Here's the drawing with two shaded views (mm, measured from the low corner). I have some questions. Coordinates: 2 decimals unless noted, no trailing zeros. Order: outer loops, then holes, each group sorted by start corner. A loop starts at its lowest first (then second) coordinate and runs counter-clockwise, first axis right, second up. Notation, with made-up numbers: (-37.75, -8) -> (-31.75, -8) arc R23 ccw to (-31.75, 8) -> close; hole circle Ø3 at (24, 89.5). An arc over 180 degrees is marked (long way). Return JSON: item names as keys, results as strings. Group by question number.
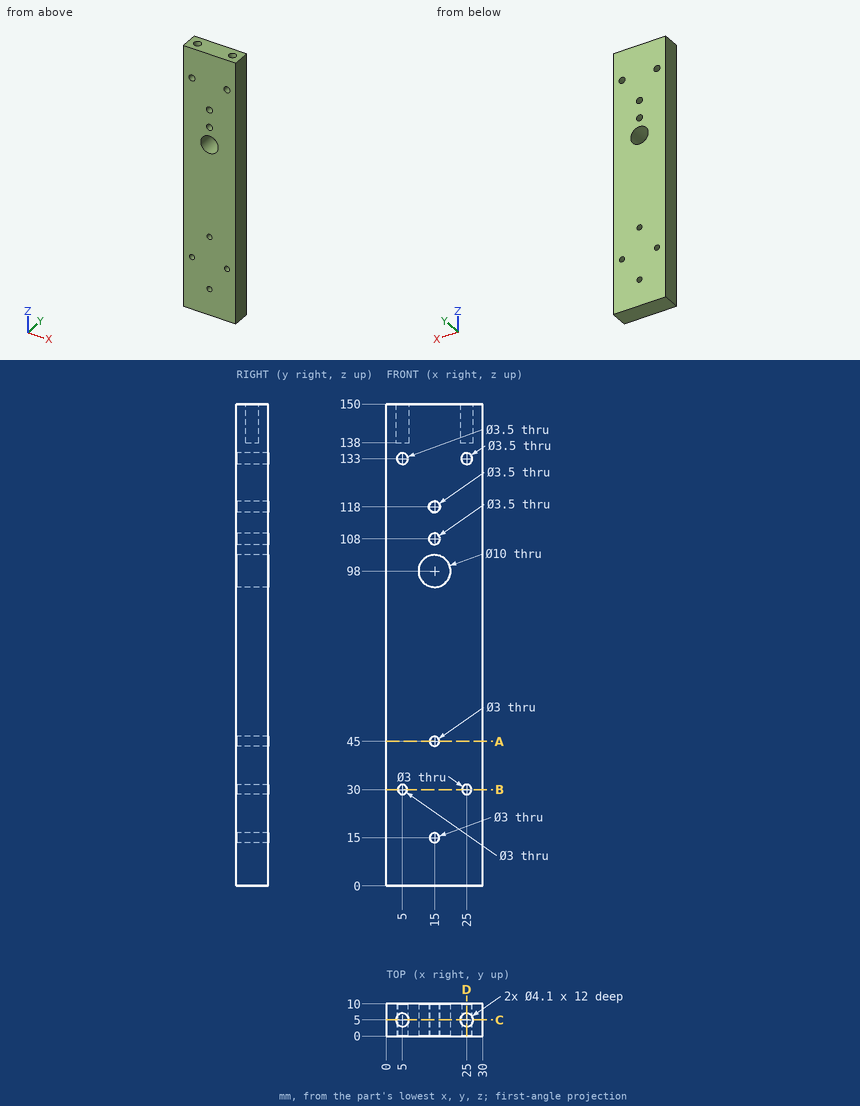
Q1. I'm going to push a flat-ended pin straight in: pin 1 Ø2 at (x, z) = (15, 118) entering from -Y. Where does the tip first touch, or does it pass through?
Q2. I need wall thicknesses on line 1 along Z through (x, y) = (15, 7.75); line 2 along X through (y, z) = (5.5, 133); line 3 along Z through (x, y) = (5, 8). Which ranges of each line are inside material? Lowest first, please. Write a range as from..to.
Q3. I want a section at A-A on z = 45. Please give me the cut outline in (x, y).
Q4. I want a section at C-C on y = 5. State how many separate pieces and enclosed holes the cut face has, and give its area (3 significant figures).
Q5. I want a section at B-B on z = 30. Please give me the cut outline in (x, y), and give its area (3 significant figures).
Q6. I want a section at D-D on x = 25. Please give me the cut outline in (y, z), and give its area (3 significant figures).
Response values:
{
 "1": {"pin 1": "passes through"},
 "2": {"line 1": "z = 0..13.5, 16.5..43.5, 46.5..93, 103..106.25, 109.75..116.25, 119.75..150", "line 2": "x = 0..3.25, 6.75..23.25, 26.75..30", "line 3": "z = 0..28.5, 31.5..131.25, 134.75..150"},
 "3": {"outline": "(0, 0) -> (13.5, 0) -> (13.5, 10) -> (0, 10) -> close; (16.5, 0) -> (30, 0) -> (30, 10) -> (16.5, 10) -> close"},
 "4": {"separate pieces": "1", "enclosed holes": "9", "area": "4,260 mm²"},
 "5": {"outline": "(0, 0) -> (3.5, 0) -> (3.5, 10) -> (0, 10) -> close; (6.5, 0) -> (23.5, 0) -> (23.5, 10) -> (6.5, 10) -> close; (26.5, 0) -> (30, 0) -> (30, 10) -> (26.5, 10) -> close", "area": "240 mm²"},
 "6": {"outline": "(0, 0) -> (10, 0) -> (10, 28.5) -> (0, 28.5) -> close; (0, 31.5) -> (10, 31.5) -> (10, 131.25) -> (0, 131.25) -> close; (0, 134.75) -> (10, 134.75) -> (10, 150) -> (7.05, 150) -> (7.05, 138) -> (2.95, 138) -> (2.95, 150) -> (0, 150) -> close", "area": "1,390 mm²"}
}
